Source: CAD feature listing. Evaluate the final solid. Frame: model axes, mm. A direction names the side the tool comes from. Round coordinates to 2 decimals unless told otherwise and drop trailing zeros. Loops run counter-clockwise (first coordinate to the right, second up) from the corner with the lowest first, then second, coordinate; pieces in that order, holes last.
Item 1: Section query B-B on z = 0. Return loops of the section in (x, y).
Item 2: Section query A-A on x = 0. Return loops of the section in (y, z).
Item 3: Pull-direction query (Z, two-part tool) for faces 1 (the flat face through (-5.5, 49, 8)), 2 (the flat face through (10, 49, 7)), 3 (the flat face through (-7, 49, -10)); classes: released by +Z, released by -Z, zero draft, split by the parting line, or undercut.
Item 4: Ray query, L1, parallel to Z at x = -7, y = 76.5; L2, parallel to Z at x = 0, y = 52.5; L3, parallel to Z at x = -5, y = 76. Return the intervals inside material, ascending.
Item 5: Access query for faces 4 (the flat face through (2, 0, -2)), 5 (the flat face through (5.25, 49.3, 4.19)), 6 (the flat face through (-3.9, 49, 0)), 7 (the flat face through (0, 49, -3.9)). Directions: +Z, -Z, +X, -X, +Y, -Y. A direction counts if a zero-diameter tool reaches every point of the face in a straight line with its end or side. Return the directions, or none.
Item 6: First-contact query: P1, Ø1, axis at y = 22.5, z = 3, coming from the +X side; P2, Ø4.5, axis at x = -0.5, y = 53.5, coming from the +Z side; P3, Ø1.7, axis at x = 0.5, y = 37, coming from the -Z side. Flat tips, straight axial feed; report the tip coordinate or a pass-through.
```python
from build123d import *

# Parameters (mm, degrees)
SKETCH_1_W      = 1.5
SKETCH_1_H      = 1.7
SKETCH_1_W_2    = 1.7
SKETCH_1_H_2    = 1.5
SKETCH_1_W_3    = 7.8
SKETCH_1_H_3    = 7.8
SKETCH_1_R      = 2.5
EXTRUDE_1_DEPTH = 100


with BuildPart() as part:
    # 草图1 → 凸台-拉伸1 (new body)
    with BuildSketch(Plane(origin=(0, 0, 0), x_dir=(1, 0, 0), z_dir=(0, 1, 0))):
        Polygon((5.5, 8.5), (5.5, 6.560660172), (5.5, 5.5), (6.560660172, 5.5), (8.5, 5.5), (10, 5.5), (10, 10), (5.5, 10), align=None)
        with Locations((9.25, 4.65)):
            Rectangle(SKETCH_1_W, SKETCH_1_H)
        Polygon((5.5, 6.560660172), (2.839339828, 3.9), (3.9, 3.9), (3.9, 2.839339828), (6.560660172, 5.5), (5.5, 5.5), align=None)
        with Locations((4.65, 9.25)):
            Rectangle(SKETCH_1_W_2, SKETCH_1_H_2)
        Rectangle(SKETCH_1_W_3, SKETCH_1_H_3)
        Circle(SKETCH_1_R, mode=Mode.SUBTRACT)
        with Locations((-4.65, 9.25)):
            Rectangle(SKETCH_1_W_2, SKETCH_1_H_2)
        Polygon((-8.5, 5.5), (-6.560660172, 5.5), (-5.5, 5.5), (-5.5, 6.560660172), (-5.5, 8.5), (-5.5, 10), (-10, 10), (-10, 5.5), align=None)
        with Locations((-9.25, 4.65)):
            Rectangle(SKETCH_1_W, SKETCH_1_H)
        Polygon((-5.5, 5.5), (-6.560660172, 5.5), (-3.9, 2.839339828), (-3.9, 3.9), (-2.839339828, 3.9), (-5.5, 6.560660172), align=None)
        Polygon((-5.5, -5.5), (-6.560660172, -5.5), (-8.5, -5.5), (-10, -5.5), (-10, -10), (-5.5, -10), (-5.5, -8.5), (-5.5, -6.560660172), align=None)
        with Locations((-4.65, -9.25)):
            Rectangle(SKETCH_1_W_2, SKETCH_1_H_2)
        with Locations((-9.25, -4.65)):
            Rectangle(SKETCH_1_W, SKETCH_1_H)
        Polygon((-3.9, -3.9), (-3.9, -2.839339828), (-6.560660172, -5.5), (-5.5, -5.5), (-5.5, -6.560660172), (-2.839339828, -3.9), align=None)
        Polygon((3.9, -3.9), (2.839339828, -3.9), (5.5, -6.560660172), (5.5, -5.5), (6.560660172, -5.5), (3.9, -2.839339828), align=None)
        Polygon((5.5, -5.5), (5.5, -6.560660172), (5.5, -8.5), (5.5, -10), (10, -10), (10, -5.5), (8.5, -5.5), (6.560660172, -5.5), align=None)
        with Locations((9.25, -4.65)):
            Rectangle(SKETCH_1_W, SKETCH_1_H)
        with Locations((4.65, -9.25)):
            Rectangle(SKETCH_1_W_2, SKETCH_1_H_2)
    extrude(amount=EXTRUDE_1_DEPTH)


solid = part.part
```
Data:
1. outline: (-3.9, 0) - (-2.5, 0) - (-2.5, 100) - (-3.9, 100) - close; (2.5, 0) - (3.9, 0) - (3.9, 100) - (2.5, 100) - close
2. outline: (0, -3.9) - (100, -3.9) - (100, -2.5) - (0, -2.5) - close; (0, 2.5) - (100, 2.5) - (100, 3.9) - (0, 3.9) - close
3. face 1: undercut
3. face 2: zero draft
3. face 3: released by -Z
4. L1: z = -10 to -5.5, 5.5 to 10
4. L2: z = -3.9 to -2.5, 2.5 to 3.9
4. L3: z = -10 to -8.5, -6.06 to -3.94, 3.94 to 6.06, 8.5 to 10
5. face 4: +Z, -Z, +X, -X, -Y
5. face 5: +Y, -Y
5. face 6: -X, +Y, -Y
5. face 7: -Z, +Y, -Y
6. P1: stops at x = 4.56
6. P2: stops at z = 3.9
6. P3: stops at z = -3.9
